```python
from build123d import *

# Parameters (mm, degrees)
EXTRUDE_1_DEPTH     = 4
SKETCH_3_R          = 2.1
CUT_EXTRUDE_1_DEPTH = 10


with BuildPart() as part:
    # 草图2 → 凸台-拉伸1 (new body)
    with BuildSketch(Plane(origin=(0, 0, 0), x_dir=(0, 0, -1), z_dir=(1, 0, 0))):
        with BuildLine():
            Line((-211.25, 80.041666667), (-157.25, 80.041666667))
            ThreePointArc((-157.25, 80.041666667), (-155.128679656, 79.16298701), (-154.25, 77.041666667))
            Line((-154.25, 77.041666667), (-154.25, 33.041666667))
            ThreePointArc((-154.25, 33.041666667), (-155.128679656, 30.920346323), (-157.25, 30.041666667))
            Line((-157.25, 30.041666667), (-161.25, 30.041666667))
            ThreePointArc((-161.25, 30.041666667), (-163.371320344, 30.920346323), (-164.25, 33.041666667))
            Line((-164.25, 33.041666667), (-164.25, 54.041666667))
            ThreePointArc((-164.25, 54.041666667), (-166.007359313, 58.284307354), (-170.25, 60.041666667))
            Line((-170.25, 60.041666667), (-211.25, 60.041666667))
            ThreePointArc((-211.25, 60.041666667), (-213.371320344, 60.920346323), (-214.25, 63.041666667))
            Line((-214.25, 63.041666667), (-214.25, 77.041666667))
            ThreePointArc((-214.25, 77.041666667), (-213.371320344, 79.16298701), (-211.25, 80.041666667))
        make_face()
    extrude(amount=EXTRUDE_1_DEPTH)

    # 草图3 → 切除-拉伸1 (cut)
    with BuildSketch(Plane(origin=(4, 0, 0), x_dir=(0, 0, -1), z_dir=(1, 0, 0))):
        with Locations((-204.25, 70.041666667)):
            Circle(SKETCH_3_R)
        with Locations((-186.25, 70.041666667)):
            Circle(SKETCH_3_R)
        with Locations((-159.25, 54.041666667)):
            Circle(SKETCH_3_R)
        with Locations((-159.25, 39.041666667)):
            Circle(SKETCH_3_R)
        with Locations((-160.25, 72.041666667)):
            Circle(SKETCH_3_R)
    extrude(amount=-CUT_EXTRUDE_1_DEPTH, mode=Mode.SUBTRACT)


solid = part.part
```
Work out the finished part from the listing and answer in its coordinate system (mm). A direction names the side the tool comes from. Give positions to 0.01 mm unless a question says otherwise; leave off trailing zeros. Loops run counter-clockwise (first coordinate to the right, second up) from the corner with the lowest first, then second, coordinate; pieces in that order, holes last. Notation, with made-up numbers: (-7.5, 77.5) -> (36.5, 77.5) arc R25 ccw to (36.5, 102.5) -> close; hole circle Ø6 at (-18, -20.5). An arc over 180 degrees is marked (long way). One line per question, with ' | ' between items. Start each with the question number.
1) Section D-D, the plane x = 1.9 is taken. Determine the outline of the cut face in (y, z), then the cut area to 3 significant figures.
2) Each of these flat-tipped pins is pushed along its axis until it touches: pin 1 (4 mm diameter, centred on y = 70.04, z = 204.25, fed in from -X); pin 2 (6.5 mm diameter, centred on y = 39.04, z = 159.25, fed in from -X); pin 3 (2 mm diameter, centred on x = 1.5, y = 40.5, fed in from +Z). Where does it stop, or does it pass through?
3) For faces 5 (the face through (2, 55, 154.25)), 6 (the face through (2, 60.042, 190)), determine the directions among +Z, -Z, +X, -X, +Y, -Y from which every point of the face is accessible in a straight line to the end or side of a thin tool.
4) Section B-B, the plane y = 40.5 is taken. Determine the outline of the cut face in (x, z), then the cut area to 3 significant figures.
5) Determine the mould class of faces 1 (the face through (2, 43, 164.25)), 2 (the face through (1.97, 30.94, 155.11)), 3 (the face through (2.03, 68.18, 185.28)), 4 (the face through (2.03, 53.24, 157.31)) for opening direction Y: +Y half, -Y half, draft (parallel to the pull), parting line (faces both ways), or undercut.
6) Section A-A, the plane z = 204.25 is taken. Determine the outline of the cut face in (x, y).
7) Straight lines are drawn through the part: L1, parallel to Y at x = 0.95, z = 204.25; L2, parallel to Y at x = 2, z = 160.25; L3, parallel to Y at x = 2.3, z = 159.25. For each, find the intervals that lie inside material, in ascending order.
8) Section C-C, the plane z = 159.25 is taken. Determine the outline of the cut face in (x, y).
Resolved:
1) outline: (30.04, 157.25) arc R3 ccw to (33.04, 154.25) -> (77.04, 154.25) arc R3 ccw to (80.04, 157.25) -> (80.04, 211.25) arc R3 ccw to (77.04, 214.25) -> (63.04, 214.25) arc R3 ccw to (60.04, 211.25) -> (60.04, 170.25) arc R6 cw to (54.04, 164.25) -> (33.04, 164.25) arc R3 ccw to (30.04, 161.25) -> close; hole circle Ø4.2 at (39.04, 159.25); hole circle Ø4.2 at (54.04, 159.25); hole circle Ø4.2 at (70.04, 186.25); hole circle Ø4.2 at (70.04, 204.25); hole circle Ø4.2 at (72.04, 160.25) | area: 1,430 mm2
2) pin 1: through | pin 2: x = 0 | pin 3: z = 164.25
3) face 5: -Z, +X, -X, +Y, -Y | face 6: +Z, +X, -X, -Y
4) outline: (0, 154.25) -> (4, 154.25) -> (4, 157.74) -> (0, 157.74) -> close; (0, 160.76) -> (4, 160.76) -> (4, 164.25) -> (0, 164.25) -> close | area: 27.9 mm2
5) face 1: draft | face 2: -Y half | face 3: undercut | face 4: undercut
6) outline: (0, 60.04) -> (4, 60.04) -> (4, 67.94) -> (0, 67.94) -> close; (0, 72.14) -> (4, 72.14) -> (4, 80.04) -> (0, 80.04) -> close
7) L1: 60.04 to 67.94, 72.14 to 80.04 | L2: 30.04 to 37.2, 40.89 to 52.2, 55.89 to 69.94, 74.14 to 80.04 | L3: 30.04 to 36.94, 41.14 to 51.94, 56.14 to 70.2, 73.89 to 80.04
8) outline: (0, 30.04) -> (4, 30.04) -> (4, 36.94) -> (0, 36.94) -> close; (0, 41.14) -> (4, 41.14) -> (4, 51.94) -> (0, 51.94) -> close; (0, 56.14) -> (4, 56.14) -> (4, 70.2) -> (0, 70.2) -> close; (0, 73.89) -> (4, 73.89) -> (4, 80.04) -> (0, 80.04) -> close
